```python
from build123d import *

# Parameters (mm, degrees)
SKETCH1_R           = 7.5
BOSS_EXTRUDE1_DEPTH = 30


with BuildPart() as part:
    # Sketch1 → Boss-Extrude1 (new body)
    with BuildSketch(Plane.XY):
        with BuildLine():
            Line((50, 0), (0, 0))
            Line((0, 0), (0, 93.284928504))
            Line((0, 93.284928504), (503.852842171, 93.284928504))
            ThreePointArc((503.852842171, 93.284928504), (518.852842171, 78.284928504), (503.852842171, 63.284928504))
            Line((503.852842171, 63.284928504), (363.350187842, 63.284928504))
            ThreePointArc((363.350187842, 63.284928504), (352.240737336, 65.393651705), (342.676664352, 71.426487861))
            ThreePointArc((342.676664352, 71.426487861), (305.687057236, 87.010211012), (267.394723934, 74.977726972))
            ThreePointArc((267.394723934, 74.977726972), (251.183228702, 66.288195069), (233.036577983, 63.284928504))
            Line((233.036577983, 63.284928504), (40, 63.284928504))
            Line((40, 63.284928504), (40, 30))
            Line((40, 30), (50, 30))
            Line((50, 30), (50, 0))
        make_face()
        with Locations((503.852842171, 78.284928504)):
            Circle(SKETCH1_R, mode=Mode.SUBTRACT)
    extrude(amount=BOSS_EXTRUDE1_DEPTH)


solid = part.part
```
Here's how the part is built. I have some questions about the finished solid (model axes, mm). A direction names the side the tool comes from. Coordinates: 2 decimals unless noted, no trailing zeros. Order: outer loops, then holes, each group sorted by start corner. A loop starts at its lowest first (then second) coordinate and runs counter-clockwise, first axis right, second up. Notation, with made-up numbers: (-39, 10) - (-25, 10) arc R25 cw to (-25, 44) - close; hole circle Ø8 at (-25.75, 28). An arc over 180 degrees is marked (long way). One line per question, with ' | ' between items. Start each with the question number.
1. If we section it at B-B (x = 222): Write out the boundary of the cut face in (y, z), and give its area (3 significant figures).
2. Please list where these lines run through material, in increasing order: line 1 along X through (y, z) = (78.5, 1.5); line 2 along Y through (x, z) = (481, 28.25); line 3 along X through (y, z) = (13, 25). Write a range as [from, to].
3. I'm going to push flat-ended pins straight in: pin 1 Ø3 at (y, z) = (53.5, 8) entering from +X; pin 2 Ø9 at (y, z) = (15.5, 14) entering from +X; pin 3 Ø8 at (x, z) = (292, 13.5) entering from -Y; pin 4 Ø12 at (x, y) = (503.85, 78.28) entering from -Z. Where does each tip first touch, or does it pass through?
4. If we section it at C-C (y = 35.5): Write out the boundary of the cut face in (x, z).
5. If we mould it in two halves opening along Y, with no side actions, what happens to faces 1 (the flat face through (40, 47, 15)), 2 (the flat face through (50, 15, 15)), 3 (the cylindrical face through (251.428, 66.372, 14.79))? For each: released by +Y, released by -Y, zero draft, split by the parting line, or undercut.
6. Which directions (+Z, -Z, +X, -X, +Y, -Y) give clear straight access to the entire face, cutting with the end or side of a thin tool? Please do faces 4 (the flat face through (25, 0, 15)), 5 (the cylindrical face through (352.389, 65.336, 14.79)), 6 (the flat face through (435, 63.285, 15)), 7 (the flat face through (45, 30, 15)), 8 (the flat face through (205, 68, 0)).
7. If we section it at A-A (z = 7.75): Write out the boundary of the cut face in (x, y).
Model answer:
1) outline: (63.28, 0) - (93.28, 0) - (93.28, 30) - (63.28, 30) - close | area: 900 mm²
2) line 1: x = [0, 272.51], [333.37, 496.36], [511.35, 518.85] | line 2: y = [63.28, 93.28] | line 3: x = [0, 50]
3) pin 1: stops at x = 40 | pin 2: stops at x = 50 | pin 3: stops at y = 85.13 | pin 4: passes through
4) outline: (0, 0) - (40, 0) - (40, 30) - (0, 30) - close
5) face 1: undercut | face 2: zero draft | face 3: released by -Y
6) face 4: +Z, -Z, +X, -X, -Y | face 5: +Z, -Z, -Y | face 6: +Z, -Z, +X, -Y | face 7: +Z, -Z, +X | face 8: -Z, +X, -X, +Y, -Y
7) outline: (0, 0) - (50, 0) - (50, 30) - (40, 30) - (40, 63.28) - (233.04, 63.28) arc R56.33 ccw to (267.39, 74.98) arc R58.27 cw to (342.68, 71.43) arc R30.32 ccw to (363.35, 63.28) - (503.85, 63.28) arc R15 ccw to (503.85, 93.28) - (0, 93.28) - close; hole circle Ø15 at (503.85, 78.28)
